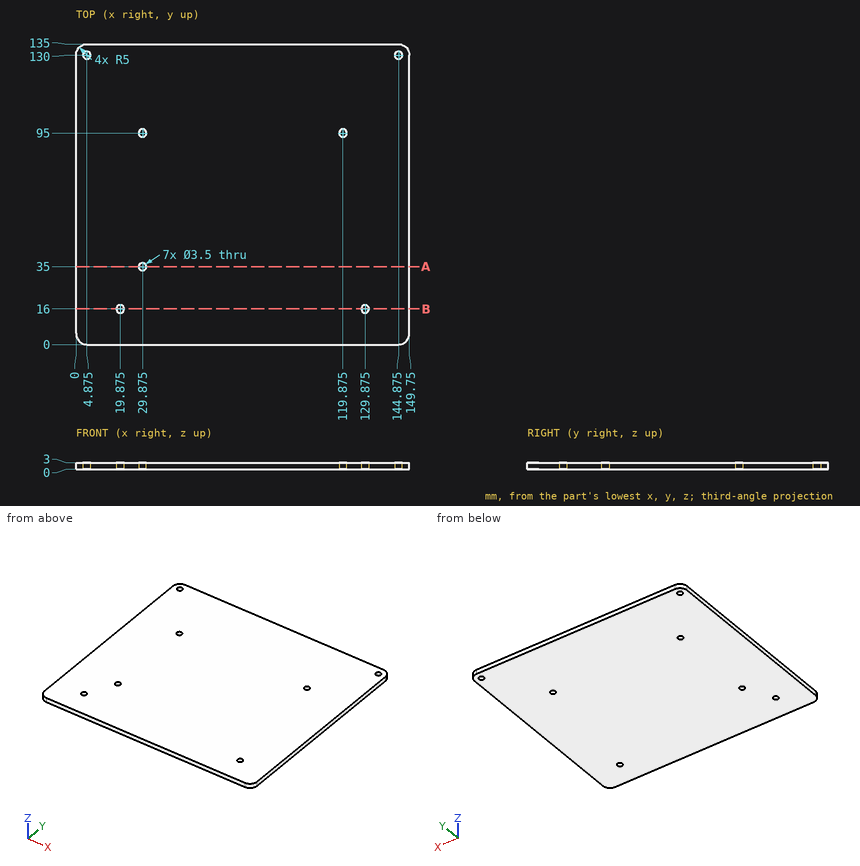
Design review of the part shown in the three views and the two pictorial views. Dimensions are in mm from the part's minimum x, y and z. Round coordinates to 2 decimals unless told otherwise and drop trailing zeros. Loops run counter-clockwise (first coordinate to the right, second up) from the corner with the lowest first, then second, coordinate; pieces in that order, holes last. Notation, with made-up numbers: (78, -3.75) - (88, -3.75) arc R32 cw to (88, 22.25) - close; hole circle Ø2 at (50.25, 59). An arc over 180 degrees is marked (long way). Answer as CSV lines item,"result".
(1) Consider section B-B on y = 16. Give the boundary of the cut face in (x, z) (3 decimals), then the cut area to 3 significant figures.
Checked values:
outline,"(0, 0) - (18.125, 0) - (18.125, 3) - (0, 3) - close; (21.625, 0) - (128.125, 0) - (128.125, 3) - (21.625, 3) - close; (131.625, 0) - (149.75, 0) - (149.75, 3) - (131.625, 3) - close"
area,"428 mm2"
(2) Wall thickness on line 1 (X direction, y = 95, z = 1.3) (3 decimals); line 2 (X direction, y = 130, z = 1.4) (3 decimals); line 3 (Y direction, x = 18.5, z = 1.3): over which ranges is each line inside the solid? List them lowest first.
Checked values:
line 1,"x = 0 to 28.125, 31.625 to 118.125, 121.625 to 149.75"
line 2,"x = 0 to 3.125, 6.625 to 143.125, 146.625 to 149.75"
line 3,"y = 0 to 14.92, 17.08 to 135"
(3) Insertion check: P1, Ø3, axis at x = 19.875, y = 16, coming from the +Z side. The pin has a flat end and moves straight along its axis. Give the tip position at first contact, or say it passes through.
Checked values:
P1,"passes through"
(4) Consider section A-A on y = 35. Give the boundary of the cut face in (x, z) (3 decimals).
Checked values:
outline,"(0, 0) - (28.125, 0) - (28.125, 3) - (0, 3) - close; (31.625, 0) - (149.75, 0) - (149.75, 3) - (31.625, 3) - close"
